Work out the finished part from the listing and answer in its coordinate system (mm). Face numbers are marked on the shaded views. Give positions to 0.01 mm unless a question says otherwise; leave off trailing zeros. Loops run counter-clockwise (first coordinate to the right, second up) from the corner with the lowest first, then second, coordinate; pieces in that order, holes last. Notation, with made-up numbers: (39.5, 35.5) - (71.5, 35.5) arc R24 cw to (71.5, 70.5) - close; hole circle Ø4 at (-4, -29). An arc over 180 degrees is marked (long way). Use one line per item in the form item = value. Start each with the question number.
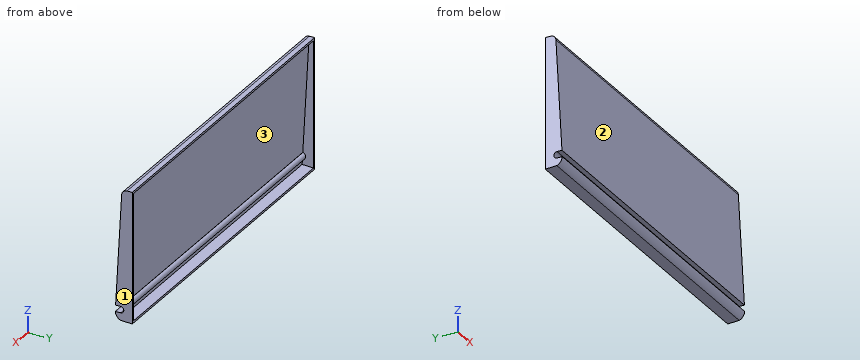
from build123d import *

# Parameters (mm, degrees)
SALIENTE_EXTRUIR1_DEPTH     = 310.007
CORTAR_EXTRUIR1_START       = 0.474917769
CORTAR_EXTRUIR1_OUTLINE_W   = 313
CORTAR_EXTRUIR1_OUTLINE_H   = 2.059275456
CORTAR_EXTRUIR1_OUTLINE_W_2 = 305.9938
CORTAR_EXTRUIR1_OUTLINE_H_2 = 118.74613036
CORTAR_EXTRUIR1_DEPTH       = 10.863473519
CORTAR_EXTRUIR2_DEPTH       = 317.143434336
SALIENTE_EXTRUIR2_REACH     = 316.176


# Read off the part's stored shape, not the designer's step: Cortar-Extruir1
with BuildPart() as part:
    # Croquis1 → Saliente-Extruir1 (new body)
    with BuildSketch(Plane(origin=(0, 0, 0), x_dir=(0, 0, -1), z_dir=(1, 0, 0))):
        with BuildLine():
            Line((-61.468, 8.001), (61.468, 8.001))
            Line((61.468, 8.001), (61.468, 0))
            ThreePointArc((61.468, 0), (58.968267477, -5.809652067), (53.031040334, -7.989113854))
            Line((53.031040334, -7.989113854), (-56.736847791, -1.999166442))
            ThreePointArc((-56.736847791, -1.999166442), (-60.09753796, -0.443275216), (-61.468, 2.9972))
            Line((-61.468, 2.9972), (-61.468, 8.001))
        make_face()
    extrude(amount=SALIENTE_EXTRUIR1_DEPTH)

    # Cortar-Extruir1 outline → Cortar-Extruir1 (cut)
    with BuildSketch(Plane(origin=(0, 0, 0), x_dir=(1, 0, 0), z_dir=(0, 0.9985144174273646, -0.054488147240394726)).offset(CORTAR_EXTRUIR1_START)):
        with Locations((155.5, 61.970362272)):
            Rectangle(CORTAR_EXTRUIR1_OUTLINE_W, CORTAR_EXTRUIR1_OUTLINE_H)
        with Locations((155.0035, -0.435959666)):
            Rectangle(CORTAR_EXTRUIR1_OUTLINE_W_2, CORTAR_EXTRUIR1_OUTLINE_H_2)
    extrude(amount=CORTAR_EXTRUIR1_DEPTH, mode=Mode.SUBTRACT)

    # Croquis3 → Cortar-Extruir2 (cut, through all)
    with BuildSketch(Plane(origin=(310.007, 0, 0), x_dir=(0, 0, -1), z_dir=(1, 0, 0))):
        with BuildLine():
            Line((47.871269455, -2.985313854), (47.871269455, -7.707549211))
            Line((47.871269455, -7.707549211), (53.031040334, -7.989113854))
            ThreePointArc((53.031040334, -7.989113854), (53.448329481, -8.000978216), (53.865669455, -7.991061486))
            Line((53.865669455, -7.991061486), (53.865669455, -2.985313854))
            ThreePointArc((53.865669455, -2.985313854), (50.868469455, 0.011886146), (47.871269455, -2.985313854))
        make_face()
    extrude(amount=-CORTAR_EXTRUIR2_DEPTH, mode=Mode.SUBTRACT)

    # Croquis4 → Saliente-Extruir2 (add, up to next)
    with BuildSketch(Plane.ZY.offset(-308.0004), mode=Mode.PRIVATE) as saliente_extruir2_sk1:
        with BuildLine():
            ThreePointArc((-54.319674223, -2.372441361), (-54.323209583, -2.4306924), (-54.313356663, -2.488212852))
            Line((-54.313356663, -2.488212852), (-53.819499619, -2.461263461))
            ThreePointArc((-53.819499619, -2.461263461), (-51.03178133, 0.007433558), (-47.991986492, -2.143260648))
            Line((-47.991986492, -2.143260648), (-47.498129447, -2.116311258))
            ThreePointArc((-47.498129447, -2.116311258), (-47.494594087, -2.058060218), (-47.504447006, -2.000539766))
            ThreePointArc((-47.504447006, -2.000539766), (-51.059461309, 0.514678882), (-54.319674223, -2.372441361))
        make_face()
    saliente_extruir2_tool1 = extrude(saliente_extruir2_sk1.sketch, amount=SALIENTE_EXTRUIR2_REACH, mode=Mode.PRIVATE) - part.part
    add(saliente_extruir2_tool1.solids().sort_by_distance((308.0004, 0.440165, -51.055395))[0])


solid = part.part
1) A cutting plane is placed at C-C (z = 52). Give the vertices of the cut face in (x, y).
2) A cutting plane is placed at A-A (x = 263.5). Give the vertices of the cut face in (y, z), plus the area to 3 significant figures.
3) Determine the mould class of the marked faces 1, 2 and 3 for opening direction X: released by +X, released by -X, zero draft, split by the parting line, or undercut.
4) A cutting plane is placed at B-B (z = 28). Give the vertices of the cut face in (x, y), plus the area to 3 significant figures.
5) Find the intervals of material crossed by probe 1 along X at (y, z) = (7, 6); probe 2 along Z at (x, y) = (262, 4.25); probe 3 along Z at (x, y) = (87, 6), in increasing order.
6) Flat-ended cylindrical pins translate along their axes: pin 1 Ø12 at (x, z) = (60, -19.5) entering from -Y; pin 2 Ø6 at (x, y) = (219, 3.5) entering from -Z; pin 3 Ø2 at (x, z) = (59.5, -7) entering from -Y. Find the tip coordinate at first contact, or state that the pin passes through.
Answer sheet:
q1.outline = (0, -2.26) - (310.01, -2.26) - (310.01, 8) - (308, 8) - (308, 3.31) - (2.01, 3.31) - (2.01, 8) - (0, 8) - close
q2.outline = (-7.99, -53.87) arc R8 ccw to (-2.85, -60.94) - (-2.85, -60.88) - (8, -61.47) - (8, -59.46) - (-2.74, -58.88) - (-2.49, -54.31) arc R0.25 ccw to (-2.37, -54.32) arc R3.51 ccw to (-2, -47.5) arc R0.25 ccw to (-2.12, -47.5) - (3.73, 59.69) - (8, 59.46) - (8, 61.47) - (3, 61.47) arc R5 ccw to (-2, 56.74) - (-7.71, -47.87) - (-2.99, -47.87) arc R3 cw to (-2.99, -53.87) - close
q2.area = 666 mm²
q3.face_1 = released by +X
q3.face_2 = zero draft
q3.face_3 = undercut
q4.outline = (0, -3.57) - (310.01, -3.57) - (310.01, 8) - (308, 8) - (308, 2) - (2.01, 2) - (2.01, 8) - (0, 8) - close
q4.area = 1,750 mm²
q5.probe_1 = 0 to 2.01, 308 to 310.01
q5.probe_2 = -61.26 to -59.26, 59.67 to 61.47
q5.probe_3 = -61.36 to -59.35, 59.57 to 61.47
q6.pin_1 = -6.49
q6.pin_2 = -61.39
q6.pin_3 = -5.53
